Here's the drawing with two shaded views (mm, measured from the low corner). I have some questions. A direction names the side the tool comes from. Coordinates: 2 decimals unless noted, no trailing zeros. Order: outer loops, then holes, each group sorted by start corner. A loop starts at its lowest first (then second) coordinate and runs counter-clockwise, first axis right, second up. Notation, with made-up numbers: (44.5, 38.25) -> (76.5, 38.25) arc R15 cw to (76.5, 65.25) -> close; hole circle Ø4 at (85, 72.25). An arc over 180 degrees is marked (long way). Write item = value, one per line.
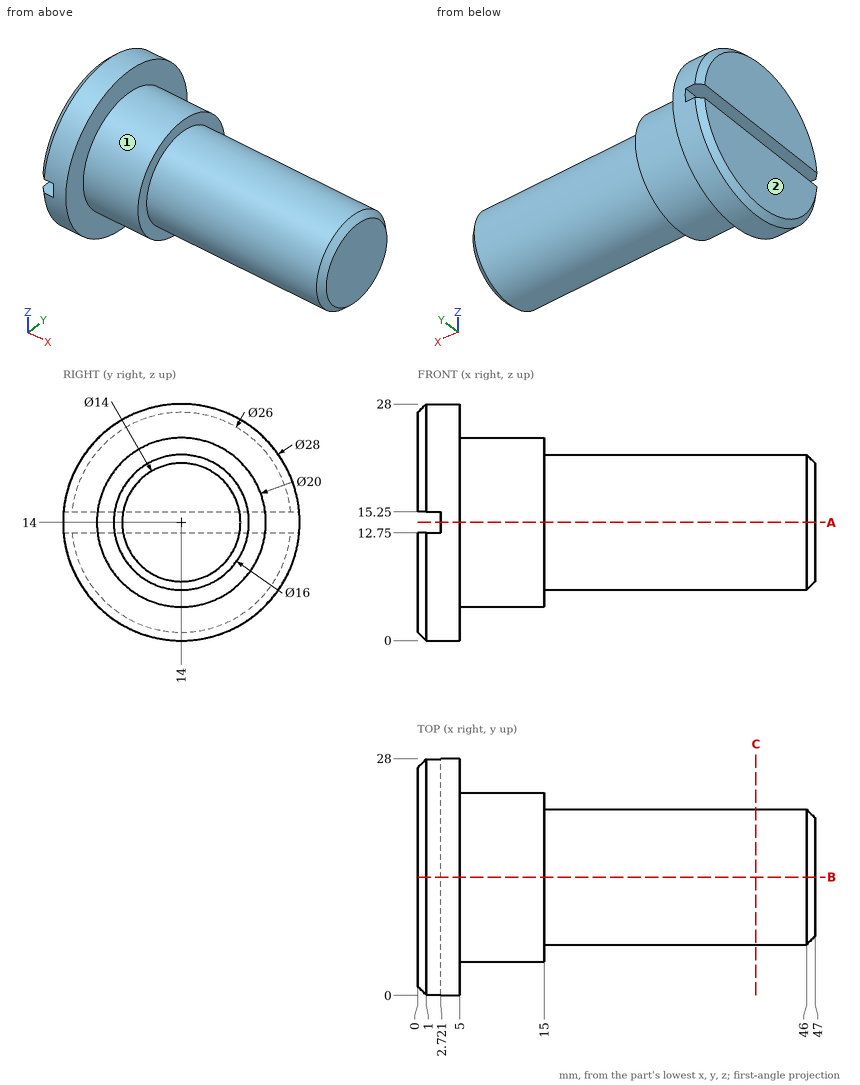
Item 1: I want a section at C-C, the plane x = 40. Please give me the cut outline in (y, z).
A:
outline = circle Ø16 at (14, 14)
Item 2: I want a section at A-A, the plane z = 14. Please give me the cut outline in (x, y).
A:
outline = (2.72, 0) -> (5, 0) -> (5, 4) -> (15, 4) -> (15, 6) -> (46, 6) -> (47, 7) -> (47, 21) -> (46, 22) -> (15, 22) -> (15, 24) -> (5, 24) -> (5, 28) -> (2.72, 28) -> close
Item 3: I want a section at B-B, the plane y = 14. Please give me the cut outline in (x, z), plus the area to 3 significant figures.
A:
outline = (0, 1) -> (1, 0) -> (5, 0) -> (5, 4) -> (15, 4) -> (15, 6) -> (46, 6) -> (47, 7) -> (47, 21) -> (46, 22) -> (15, 22) -> (15, 24) -> (5, 24) -> (5, 28) -> (1, 28) -> (0, 27) -> (0, 15.25) -> (2.72, 15.25) -> (2.72, 12.75) -> (0, 12.75) -> close
area = 843 mm2
Item 4: If I drill on probe 1 along X at (y, z) = (20.5, 21); probe 2 along X at (y, z) = (14.5, 15); probe 3 along Z at (x, y) = (10.5, 14), over which ranges is the centre line in solid material (lowest first)?
A:
probe_1 = 0 to 15
probe_2 = 2.72 to 47
probe_3 = 4 to 24
Item 5: For the marked faces 1 and 2, which set-ups out of +Z, -Z, +X, -X, +Y, -Y let a thin tool reach every point of the face, with its end or its side?
A:
face_1 = +X
face_2 = +Z, -Z, -X, +Y, -Y
Item 6: I'm going to push flat-ended pins straight in: P1, Ø3, axis at x = 2, y = 19.5, coming from the -Z side; P2, Ø6, axis at x = 11, y = 4.5, coming from the +Z side; P3, Ø3, axis at x = 1, y = 17, coming from the +Z side; P4, Ø3, axis at y = 15, z = 22, coming from the +X side. Where does each tip first touch, or does it pass through?
A:
P1 = 0.58
P2 = 21.6
P3 = 27.92
P4 = 47
